```python
from build123d import *

# Parameters (mm, degrees)
BOSS_EXTRUDE1_DEPTH     = 52
FILLET1_R               = 1
SHELL1_T                = -2
SKETCH2_R               = 9
SKETCH2_R_2             = 4
BOSS_EXTRUDE2_DEPTH     = 2.5
SKETCH3_R               = 14.5
CUT_EXTRUDE1_DEPTH      = 195.753690594
CUT_EXTRUDE2_DEPTH      = 153.410629551
CUT_EXTRUDE2_DEPTH_BACK = 153.410629551
SKETCH4_R               = 14.5


with BuildPart() as part:
    # Sketch1 → Boss-Extrude1 (new body)
    with BuildSketch(Plane(origin=(0, 0, 0), x_dir=(1, 0, 0), z_dir=(0, 1, 0))):
        with BuildLine():
            Line((125, -62), (125, 62))
            ThreePointArc((125, 62), (122.656854249, 67.656854249), (117, 70))
            Line((117, 70), (-117, 70))
            ThreePointArc((-117, 70), (-122.656854249, 67.656854249), (-125, 62))
            Line((-125, 62), (-125, -62))
            ThreePointArc((-125, -62), (-122.656854249, -67.656854249), (-117, -70))
            Line((-117, -70), (117, -70))
            ThreePointArc((117, -70), (122.656854249, -67.656854249), (125, -62))
        make_face()
    extrude(amount=BOSS_EXTRUDE1_DEPTH)

    # Fillet1
    fillet1_edges = [part.edges().sort_by_distance(p)[0] for p in [
        (0, 0, -70),
        (122.656854249, 0, -67.656854249),
        (125, 0, 0),
        (122.656854249, 0, 67.656854249),
        (0, 0, 70),
        (-122.656854249, 0, 67.656854249),
        (-125, 0, 0),
        (-122.656854249, 0, -67.656854249),
    ]]
    fillet(fillet1_edges, radius=FILLET1_R)

    # Shell1
    shell1_openings = [part.faces().sort_by_distance(p)[0] for p in [
        (0, 52, 0),
    ]]
    offset(amount=SHELL1_T, openings=shell1_openings, kind=Kind.INTERSECTION)

    # Sketch2 → Boss-Extrude2 (add)
    # profile 1 of 4: a face of its own
    with BuildSketch(Plane.XZ):
        with Locations(Location((76, 51, 0), (0, 0, 90))):
            Circle(SKETCH2_R)
        with Locations(Location((76, 51, 0), (0, 0, 270))):
            Circle(SKETCH2_R_2, mode=Mode.SUBTRACT)
    # profile 2 of 4: a face of its own
    with BuildSketch(Plane.XZ):
        with Locations(Location((76, -51, 0), (0, 0, 90))):
            Circle(SKETCH2_R)
        with Locations(Location((76, -51, 0), (0, 0, 90))):
            Circle(SKETCH2_R_2, mode=Mode.SUBTRACT)
    # profile 3 of 4: a face of its own
    with BuildSketch(Plane.XZ):
        with Locations(Location((-76, -51, 0), (0, 0, 90))):
            Circle(SKETCH2_R)
        with Locations(Location((-76, -51, 0), (0, 0, 270))):
            Circle(SKETCH2_R_2, mode=Mode.SUBTRACT)
    # profile 4 of 4: a face of its own
    with BuildSketch(Plane.XZ):
        with Locations(Location((-76, 51, 0), (0, 0, 90))):
            Circle(SKETCH2_R)
        with Locations(Location((-76, 51, 0), (0, 0, 90))):
            Circle(SKETCH2_R_2, mode=Mode.SUBTRACT)
    extrude(amount=BOSS_EXTRUDE2_DEPTH)

    # Sketch3 → Cut-Extrude1 (cut, through all)
    with BuildSketch(Plane(origin=(0, 0, -70), x_dir=(-1, 0, 0), z_dir=(0, 0, -1))):
        with Locations((-55, 25.3)):
            Circle(SKETCH3_R)
        with Locations((0, 25.3)):
            Circle(SKETCH3_R)
        with Locations((55, 25.3)):
            Circle(SKETCH3_R)
    extrude(amount=-CUT_EXTRUDE1_DEPTH, mode=Mode.SUBTRACT)

    # Sketch4 → Cut-Extrude2 (cut, two sides: drawn at the far end of the back side and taken through both)
    with BuildSketch(Plane(origin=(0, 0, 0), x_dir=(0, 0, -1), z_dir=(1, 0, 0)).offset(-CUT_EXTRUDE2_DEPTH_BACK)):
        with Locations((31, 25.3)):
            Circle(SKETCH4_R)
        with Locations(Location((-31, 25.3, 0), (0, 0, 180))):
            Circle(SKETCH4_R)
    extrude(amount=CUT_EXTRUDE2_DEPTH + CUT_EXTRUDE2_DEPTH_BACK, mode=Mode.SUBTRACT)


solid = part.part
```
The model under review builds one solid part; all positions refer to its coordinate system, in mm. A direction names the side the tool comes from. Give positions to 0.01 mm unless a question says otherwise; leave off trailing zeros. Order: outer loops, then holes, each group sorted by start corner. A loop starts at its lowest first (then second) coordinate and runs counter-clockwise, first axis right, second up. Notation, with made-up numbers: (20, 15) - (44, 15) arc R21 ccw to (44, 33) - close; hole circle Ø4 at (36.25, 60.25). An arc over 180 degrees is marked (long way). Use CSV: the item, a comma, the result in double quotes. Start each with the question number.
Q1. Clearance check with flat-ended pins moving along their axes: pin 1 Ø2.5 at (x, z) = (-74.5, 52) entering from -Y; pin 2 Ø17.5 at (x, y) = (55, 25.3) entering from +Z; pin 3 Ø3 at (x, z) = (-45, -17) entering from +Y. State where each tip first meets the part, or that it passes through.
Q2. We need section C-C, the plane y = 46.5. Write out the cut boundary in (x, z), and give its area (3 significant figures).
Q3. We need section B-B, the plane z = 31. Write out the cut boundary in (x, y), and give its area (3 significant figures).
Q4. The part is to be moulded in two halves that separate along Y. For faces 1 (the cylindrical face through (122.594, 26.143, 67.719)), 2 (the flat face through (-74, -2.5, -47)), 3 (the cylindrical face through (123.99, 20.94, 44.83)), say which applies: +Y half, -Y half, draft (parallel to the pull), parting line (faces both ways), or undercut.
Q5. We need section A-A, the plane x = 0. Write out the cut boundary in (y, z).
Q6. We need section D-D, the plane x = 35.5. Write out the cut boundary in (y, z), and give its area (3 significant figures).
Q7. To check wall thickness, follow line 1 along X through (y, z) = (-1.75, -51); line 2 along X through (y, z) = (8, 21.5); line 3 along Z through (x, y) = (90, 3). State the ranges of each line that lie inside material, in increasing order. Write a range as [from, to].
Q8. Tool access review of faces 4 (the flat face through (2, 43, -70)), 5 (the cylindrical face through (-67.214, -1.232, -52.951)), 6 (the flat face through (123, 27, 1)): name each direction out of +Z, -Z, +X, -X, +Y, -Y from which nothing blocks a thin tool from reaching the whole face with its end or side.
Outcome:
1,pin 1,"stops at y = 0"
1,pin 2,"passes through"
1,pin 3,"stops at y = 2"
2,outline,"(-125, -62) arc R8 ccw to (-117, -70) - (117, -70) arc R8 ccw to (125, -62) - (125, 62) arc R8 ccw to (117, 70) - (-117, 70) arc R8 ccw to (-125, 62) - close; hole (-123, -62) arc R6 ccw to (-117, -68) - (117, -68) arc R6 ccw to (123, -62) - (123, 62) arc R6 ccw to (117, 68) - (-117, 68) arc R6 ccw to (-123, 62) - close"
2,area,"1,520 mm^2"
3,outline,"(-125, 1) arc R1 ccw to (-124, 0) - (124, 0) arc R1 ccw to (125, 1) - (125, 10.8) - (123, 10.8) - (123, 2) - (-123, 2) - (-123, 10.8) - (-125, 10.8) - close; (-125, 39.8) - (-123, 39.8) - (-123, 52) - (-125, 52) - close; (123, 39.8) - (125, 39.8) - (125, 52) - (123, 52) - close"
3,area,"584 mm^2"
4,face 1,"draft"
4,face 2,"-Y half"
4,face 3,"undercut"
5,outline,"(0, -69) arc R1 ccw to (1, -70) - (10.8, -70) - (10.8, -68) - (2, -68) - (2, 68) - (10.8, 68) - (10.8, 70) - (1, 70) arc R1 ccw to (0, 69) - close; (39.8, -70) - (52, -70) - (52, -68) - (39.8, -68) - close; (39.8, 68) - (52, 68) - (52, 70) - (39.8, 70) - close"
6,outline,"(0, -69) arc R1 ccw to (1, -70) - (52, -70) - (52, -68) - (2, -68) - (2, 68) - (52, 68) - (52, 70) - (1, 70) arc R1 ccw to (0, 69) - close"
6,area,"480 mm^2"
7,line 1,"x = [-85, -80], [-72, -67], [67, 72], [80, 85]"
7,line 2,"x = [-125, -123], [123, 125]"
7,line 3,"z = [-70, -68], [68, 70]"
8,face 4,"-Z, +X, -X, +Y, -Y"
8,face 5,"-Y"
8,face 6,"+Y"
